Design review of the part built by this model. Coordinates are the model's own, in mm. Face numbers are marked on the shaded views. Round coordinates to 2 decimals unless told otherwise and drop trailing zeros. Write each loop counter-clockwise with the first axis right and the second up, starting at its lowest first coordinate (ties: lowest second). Pieces come first, ordered by that corner, then holes. Notation, with made-up numbers: M -29.75,50 L -25.75,50 A37 ccw -25.75,87 Z; hole C -6.75,75 d6. An arc over 180 degrees is marked long. Use CSV: the item, a comma, the result in double quotes.
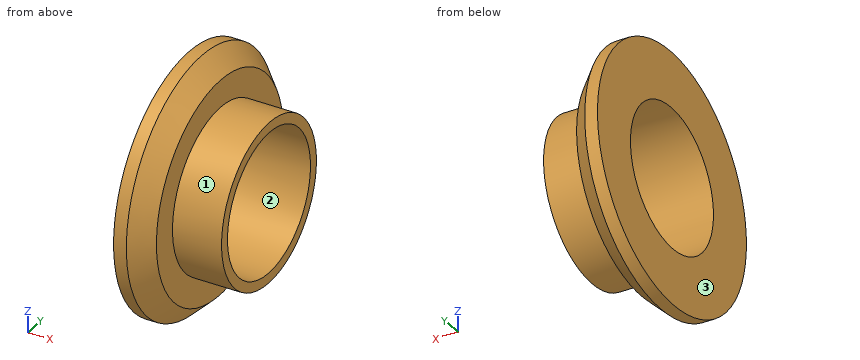
from build123d import *


with BuildPart() as part:
    # Axial profile (mm) → Full revolution (revolve)
    with BuildSketch(Plane.XY, mode=Mode.PRIVATE) as full_revolution_sk:
        Polygon((1, 11.1125), (13.7, 11.1125), (13.7, 12.7), (6, 12.7), (6, 17), (3, 19.94), (1, 19.94), align=None)
    revolve(full_revolution_sk.sketch.rotate(Axis((-110, 0, 0), (1, 0, 0)), 90), axis=Axis((-110, 0, 0), (1, 0, 0)))


solid = part.part
1) The part is to be moulded in two halves that separate along Z. For the marked faces 1, 2 and 3, say which applies: released by +Z, released by -Z, zero draft, split by the parting line, or undercut.
Answers:
face 1,"split by the parting line"
face 2,"undercut"
face 3,"zero draft"
2) Add section C-C on x = 12.5. Write out the cut boundary in (y, z) (1 decimal).
Answers:
outline,"C 0,0 d25.4; hole C 0,0 d22.2"
3) Wall thickness on line 1 along Y through (x, z) = (7.5, 0); line 2 along X through (y, z) = (5.5, -15); line 3 along Y through (x, z) = (5.25, -1.5): over which ranges is each line inside the solid? List them lowest first. Write a range as [from, to].
Answers:
line 1,"[-12.7, -11.11], [11.11, 12.7]"
line 2,"[1, 6]"
line 3,"[-17.67, -11.01], [11.01, 17.67]"
4) For pin 1 Ø1 at (x, z) = (4.5, -6) entering from -Y; pin 2 Ø1 at (x, z) = (5.5, -4.5) entering from -Y; pin 3 Ø5 at (x, z) = (7.5, 3.5) entering from -Y, all flat-tipped, find the tip position at first contact; note any pin that passes through.
Answers:
pin 1,"y = -18.01"
pin 2,"y = -17.42"
pin 3,"y = -17.68"
5) Add section A-A on y = 0. Write out the cut boundary in (x, z).
Answers:
outline,"M 1,-19.94 L 3,-19.94 L 6,-17 L 6,-12.7 L 13.7,-12.7 L 13.7,-11.11 L 1,-11.11 Z; M 1,11.11 L 13.7,11.11 L 13.7,12.7 L 6,12.7 L 6,17 L 3,19.94 L 1,19.94 Z"
